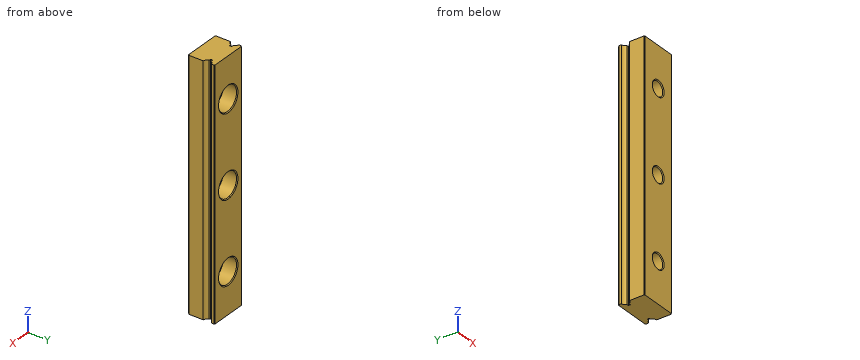
```python
from build123d import *

# Parameters (mm, degrees)
EXTRUDE1_DEPTH             = 60
EXTRUDE2_REACH             = 62.519
SKETCH2_R                  = 1.75
SKETCH_R                   = 3
SKETCH_R_2                 = 1.75
EXTRUDE4_DEPTH             = 3.5
CHAMFER1_SIZE              = 0.2
LPATTERN1_COUNT            = 3
LPATTERN1_PITCH            = 20
CHAMFER1_OF_LPATTERN1_SIZE = 0.2


with BuildPart() as part:
    # Sketch1 → Extrude1 (new body)
    with BuildSketch(Plane.XY):
        with BuildLine():
            Line((-4.3, -3.25), (4.3, -3.25))
            Line((4.3, -3.25), (4.5, -3.05))
            Line((4.5, -3.05), (4.5, 0.455012563))
            ThreePointArc((4.5, 0.455012563), (3.924845827, 0.712323349), (3.617735397, 1.2625))
            Line((3.617735397, 1.2625), (3.15008224, 1.2625))
            Line((3.15008224, 1.2625), (3.15008224, 1.7625))
            Line((3.15008224, 1.7625), (3.65008224, 1.7625))
            ThreePointArc((3.65008224, 1.7625), (3.973877727, 2.229724887), (4.5, 2.444987437))
            Line((4.5, 2.444987437), (4.5, 3.05))
            Line((4.5, 3.05), (4.3, 3.25))
            Line((4.3, 3.25), (-4.3, 3.25))
            Line((-4.3, 3.25), (-4.5, 3.05))
            Line((-4.5, 3.05), (-4.5, 2.444987437))
            ThreePointArc((-4.5, 2.444987437), (-3.973877727, 2.229724887), (-3.65008224, 1.7625))
            Line((-3.65008224, 1.7625), (-3.15008224, 1.7625))
            Line((-3.15008224, 1.7625), (-3.15008224, 1.2625))
            Line((-3.15008224, 1.2625), (-3.617735397, 1.2625))
            ThreePointArc((-3.617735397, 1.2625), (-3.924845827, 0.712323349), (-4.5, 0.455012563))
            Line((-4.5, 0.455012563), (-4.5, -3.05))
            Line((-4.5, -3.05), (-4.3, -3.25))
        make_face()
    extrude(amount=EXTRUDE1_DEPTH)

    # Sketch2 → Extrude2 (cut, up to next)
    with BuildSketch(Plane(origin=(0, 3.25, 0), x_dir=(1, 0, 0), z_dir=(0, 1, 0)), mode=Mode.PRIVATE) as extrude2_sk1:
        with Locations(Location((0, -10, 0), (0, 0, 270))):
            Circle(SKETCH2_R)
    extrude2_tool1 = extrude(extrude2_sk1.sketch, amount=-EXTRUDE2_REACH, mode=Mode.PRIVATE) & part.part
    extrude2 = extrude2_tool1.solids().sort_by_distance((0, 3.25, 10))[0]
    add(extrude2, mode=Mode.SUBTRACT)

    # Sketch → Extrude4 (cut)
    with BuildSketch(Plane(origin=(0, 3.25, 0), x_dir=(1, 0, 0), z_dir=(0, 1, 0))):
        with Locations(Location((0, -10, 0), (0, 0, 270))):
            Circle(SKETCH_R)
        with Locations(Location((0, -10, 0), (0, 0, 270))):
            Circle(SKETCH_R_2, mode=Mode.SUBTRACT)
    extrude4 = extrude(amount=-EXTRUDE4_DEPTH, mode=Mode.SUBTRACT)

    # Chamfer1
    chamfer1_edges = [part.edges().sort_by_distance(p)[0] for p in [
        (0, -3.25, 8.25),
        (0, 3.25, 7),
    ]]
    chamfer(chamfer1_edges, length=CHAMFER1_SIZE)

    # LPattern1: Extrude2, Extrude4 ×3
    with Locations(*[(0, 0, i * LPATTERN1_PITCH) for i in range(1, LPATTERN1_COUNT)]):
        add(extrude2, mode=Mode.SUBTRACT)
        add(extrude4, mode=Mode.SUBTRACT)

    # Chamfer1 of LPattern1
    chamfer1_of_lpattern1_edges = [part.edges().sort_by_distance(p)[0] for p in [
        (0, -3.25, 28.25),
        (0, 3.25, 27),
        (0, -3.25, 48.25),
        (0, 3.25, 47),
    ]]
    chamfer(chamfer1_of_lpattern1_edges, length=CHAMFER1_OF_LPATTERN1_SIZE)


solid = part.part
```
Build history of the part. All positions in model axes, mm. Round coordinates to 2 decimals unless told otherwise and drop trailing zeros. Order: outer loops, then holes, each group sorted by start corner. A loop starts at its lowest first (then second) coordinate and runs counter-clockwise, first axis right, second up. Notation, with made-up numbers: (-13.75, 78.25) -> (-2.75, 78.25) arc R32 cw to (-2.75, 114.25) -> close; hole circle Ø3 at (33, -27.5). An arc over 180 degrees is marked (long way). Answer in a Markdown table with one row per item.
1) Band-saw the part on B-B on z = 45. Give the cut face in (x, y).
Values:
| item | result |
|---|---|
| outline | (-4.5, -3.05) -> (-4.3, -3.25) -> (4.3, -3.25) -> (4.5, -3.05) -> (4.5, 0.46) arc R1 cw to (3.62, 1.26) -> (3.15, 1.26) -> (3.15, 1.76) -> (3.65, 1.76) arc R1 cw to (4.5, 2.44) -> (4.5, 3.05) -> (4.3, 3.25) -> (-4.3, 3.25) -> (-4.5, 3.05) -> (-4.5, 2.44) arc R1 cw to (-3.65, 1.76) -> (-3.15, 1.76) -> (-3.15, 1.26) -> (-3.62, 1.26) arc R1 cw to (-4.5, 0.46) -> close |
2) Pin check, flat tip, straight feed: P1, Ø3, axis at x = 0.5, z = 29, coming from the +Y side. Stop position of the tip, or through.
Values:
| item | result |
|---|---|
| P1 | y = -0.25 |
3) Wall check: L1, parallel to X at y = -1.1, z = 10; L2, parallel to Y at x = 3.5, z = 39; L3, parallel to Z at x = 0.5, y = -2.75. Give the ranges that are in metal, low to high.
Values:
| item | result |
|---|---|
| L1 | -4.5 to -1.75, 1.75 to 4.5 |
| L2 | -3.25 to 1.26, 1.76 to 3.25 |
| L3 | 0 to 8.32, 11.68 to 28.32, 31.68 to 48.32, 51.68 to 60 |
4) Band-saw the part on C-C on x = 0. Give the number of separate pieces and of enclosed holes in the cut face, and give its area (3 significant figures).
Values:
| item | result |
|---|---|
| separate pieces | 4 |
| enclosed holes | 0 |
| area | 295 mm2 |
